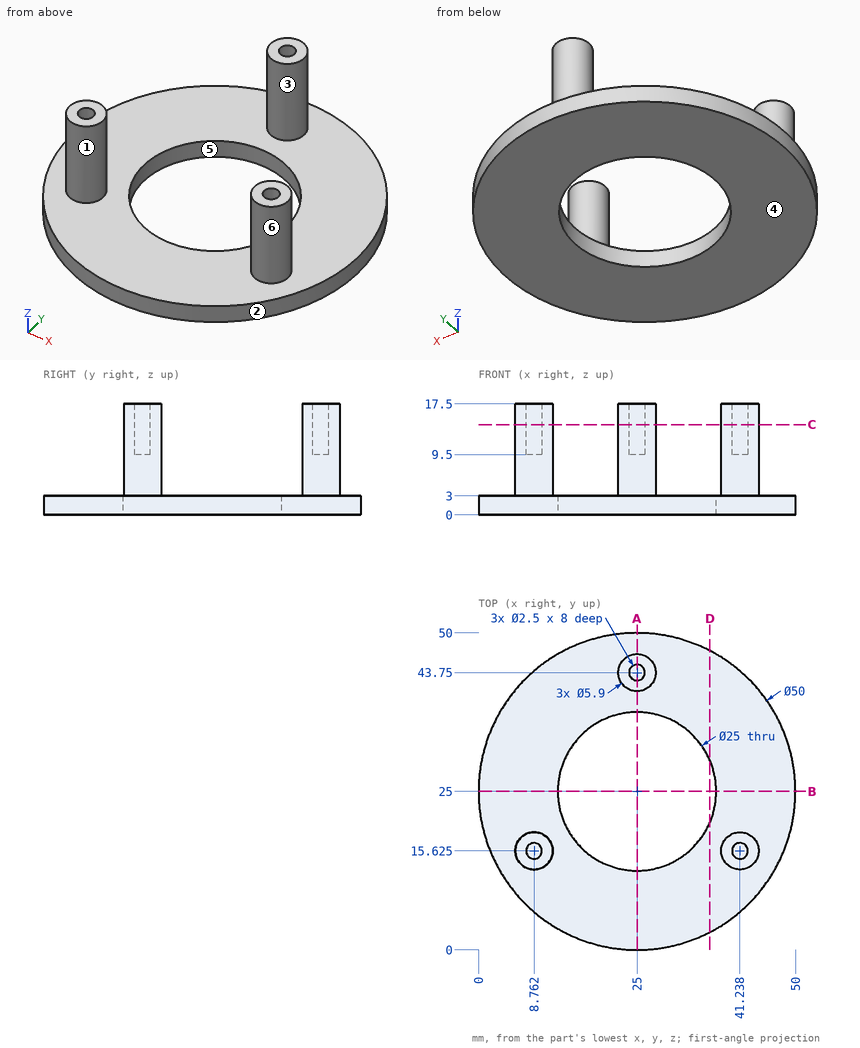
Geometry check sheet. Reference: drawing and pictorial views, mm from the part's lowest x, y, z. A direction names the side the tool comes from. Give positions to 0.01 mm unless a question says otherwise; leave off trailing zeros. Order: outer loops, then holes, each group sorted by start corner. A loop starts at its lowest first (then second) coordinate and runs counter-clockwise, first axis right, second up. Notation, with made-up numbers: M 57.5,16.25 L 65.5,16.25 A32 ccw 65.5,53.25 Z; hole C 22.25,36.5 d3. An arc over 180 degrees is marked long. Answer as a JSON object with one key per item and string values. Group by question number.
1) Access from +Z, -Z, +X, -X, +Y, -Y to the whole of each face (thin tool, end or side, straight path). Record for the marked faces 1 and 2.
2) Cross-section at A-A (x = 25). Enter the section's corners in (y, z).
3) Cross-section at B-B (y = 25). Enter the section's corners in (x, z), then the cut area to 3 significant figures.
4) Cross-section at D-D (x = 36.5). Enter the section's corners in (y, z), then the cut area to 3 significant figures.
5) Cross-section at C-C (z = 14.25). Enter the section's corners in (x, y) (3 decimals).
6) Scan lines: line 1 along Y through (x, z) = (25, 1.85); line 2 along Y through (x, z) = (25, 13.5); line 3 along Z through (x, y) = (38, 36). Record each from-to range of solid material in increasing order. Write a range as [from, to].
7) Mould release check, pull along X, two halves, no side actions. Record for the marked faces 3, 4, 5 and 6: released by +X, released by -X, zero draft, split by the parting line, or undercut.
8) Depth check by flat-ended pin: pin 1 Ø10 at (x, y) = (9.5, 16.5) entering from -Z; pin 2 Ø2 at (x, y) = (8.76, 15.62) entering from +Z; pin 3 Ø3 at (x, y) = (39.5, 43.5) entering from +Z; pin 4 Ø5 at (x, z) = (26.5, 11) entering from -Y. Enter the tip coordinate at first touch or a pass-through.
Result sheet:
{
 "1": {"face 1": "+Z", "face 2": "+Z, -Z"},
 "2": {"outline": "M 0,0 L 12.5,0 L 12.5,3 L 0,3 Z; M 37.5,0 L 50,0 L 50,3 L 46.7,3 L 46.7,17.5 L 45,17.5 L 45,9.5 L 42.5,9.5 L 42.5,17.5 L 40.8,17.5 L 40.8,3 L 37.5,3 Z"},
 "3": {"outline": "M 0,0 L 12.5,0 L 12.5,3 L 0,3 Z; M 37.5,0 L 50,0 L 50,3 L 37.5,3 Z", "area": "75.0 mm2"},
 "4": {"outline": "M 2.8,0 L 20.1,0 L 20.1,3 L 2.8,3 Z; M 29.9,0 L 47.2,0 L 47.2,3 L 29.9,3 Z", "area": "104 mm2"},
 "5": {"outline": "C 8.762,15.625 d5.9; C 25,43.75 d5.9; C 41.238,15.625 d5.9; hole C 8.762,15.625 d2.5; hole C 25,43.75 d2.5; hole C 41.238,15.625 d2.5"},
 "6": {"line 1": "y = [0, 12.5], [37.5, 50]", "line 2": "y = [40.8, 42.5], [45, 46.7]", "line 3": "z = [0, 3]"},
 "7": {"face 3": "split by the parting line", "face 4": "zero draft", "face 5": "undercut", "face 6": "undercut"},
 "8": {"pin 1": "stops at z = 0", "pin 2": "stops at z = 9.5", "pin 3": "stops at z = 3", "pin 4": "stops at y = 40.8"}
}
